Could you check a few things on this model? Use its own coordinates, in mm. Face numbers are marked on the shaded views. Round coordinates to 2 decimals unless told otherwise and drop trailing zeros. Loops run counter-clockwise (first coordinate to the right, second up) from the corner with the lowest first, then second, coordinate; pieces in that order, holes last. Notation, with made-up numbers: (-18, 69.5) -> (36, 69.5) arc R21 ccw to (36, 97.5) -> close; hole circle Ø4 at (-28, 71). An arc over 180 degrees is marked (long way). Put each result on its own line as item: value. Start each with the question number.
1. I need wall thicknesses on line 1 (Y direction, x = 0, z = 0); line 2 (X direction, y = 7.5, z = 0.75); line 3 (Z direction, x = 2, y = 13.75). Which ranges of each line are inside material? Lowest first, please. Write a range as [from, to].
2. Imagine slicing it at B-B, the plane y = 11.5. Please give me the cut outline in (x, z).
3. If we mould it in two halves opening along X, with no side actions, what happens to the marked faces 1, 2 and 3? For each: pulls with the +X half, pulls with the -X half, needs draft (parallel to the pull), parting line crosses it, or undercut.
4. Imagine slicing it at A-A, the plane z = 0. Please give me the cut outline in (x, y), and give its area (3 significant figures).
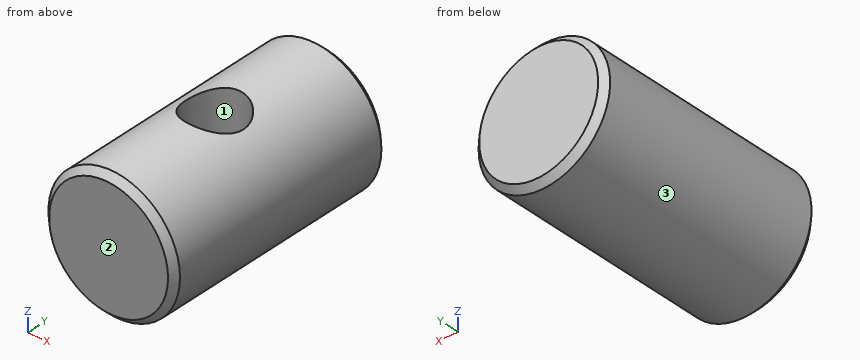
```python
from build123d import *

# Parameters (mm, degrees)
SKETCH1_R                           = 3.9624
BOSS_EXTRUDE1_DEPTH                 = 14.351
CHAMFER1_SIZE                       = 0.381
F_9_64_0_14063_DIAMETER_HOLE3_D     = 3.4544
F_9_64_0_14063_DIAMETER_HOLE3_DEPTH = 6.35
F_9_64_0_14063_DIAMETER_HOLE3_TIP   = 1.037806461


with BuildPart() as part:
    # Sketch1 → Boss-Extrude1 (new body)
    with BuildSketch(Plane(origin=(0, 0, 0), x_dir=(1, 0, 0), z_dir=(0, 1, 0))):
        Circle(SKETCH1_R)
    extrude(amount=BOSS_EXTRUDE1_DEPTH)

    # Chamfer1
    chamfer1_edges = [part.edges().sort_by_distance(p)[0] for p in [
        (-3.9624, 0, 0),
        (-3.9624, 14.351, 0),
    ]]
    chamfer(chamfer1_edges, length=CHAMFER1_SIZE)

    # 9/64 (0.14063) Diameter Hole3
    with Locations(Plane.XY.offset(3.96875)):
        with Locations((0, 7.1628)):
            Hole(F_9_64_0_14063_DIAMETER_HOLE3_D / 2, depth=F_9_64_0_14063_DIAMETER_HOLE3_DEPTH)
            with Locations((0, 0, -(F_9_64_0_14063_DIAMETER_HOLE3_DEPTH + F_9_64_0_14063_DIAMETER_HOLE3_TIP / 2))):  # 118° drill point
                Cone(0, F_9_64_0_14063_DIAMETER_HOLE3_D / 2, F_9_64_0_14063_DIAMETER_HOLE3_TIP, mode=Mode.SUBTRACT)


solid = part.part
```
Entries:
1. line 1: [0, 5.44], [8.89, 14.35]
1. line 2: [-3.89, -1.69], [1.69, 3.89]
1. line 3: [-3.42, 3.42]
2. outline: circle Ø7.92 at (0, 0)
3. face 1: undercut
3. face 2: needs draft
3. face 3: parting line crosses it
4. outline: (-3.96, 0.38) -> (-3.58, 0) -> (3.58, 0) -> (3.96, 0.38) -> (3.96, 13.97) -> (3.58, 14.35) -> (-3.58, 14.35) -> (-3.96, 13.97) -> close; hole circle Ø3.45 at (0, 7.16)
4. area: 104 mm^2
